Geometry check sheet. Reference: the model listing, model coordinates, mm. A direction names the side the tool comes from. Round coordinates to 2 decimals unless told otherwise and drop trailing zeros. Order: outer loops, then holes, each group sorted by start corner. A loop starts at its lowest first (then second) coordinate and runs counter-clockwise, first axis right, second up. Notation, with made-up numbers: (51, 5.25) - (62, 5.25) arc R32 cw to (62, 39.25) - close; hole circle Ø8 at (46, -2). An arc over 180 degrees is marked (long way). Write each question's results on one line, items separated by ' | '.
Autodesk Inventor part; units mm, degrees
ref_plane "YZ Plane" through (0, 0, 0) normal (1, 0, 0) x (0, 1, 0)
ref_plane "XZ Plane" through (0, 0, 0) normal (0, 1, 0) x (-1, 0, 0)
ref_plane "XY Plane" through (0, 0, 0) normal (0, 0, 1) x (1, 0, 0)
sketch "Sketch1" plane through (0, 0, 0) normal (0, 0, 1) x (1, 0, 0)
  circle A0 centre (0, 0) radius 1
  dimension "d0" = 2
extrude "Extrusion1" add sketch "Sketch1" along normal blind 30
ref_plane "Work Plane1" through (0, 0, 23) normal (0, 0, 1) x (1, 0, 0)
ref_plane "Work Plane2" through (0, 0, 7) normal (0, 0, -1) x (-1, 0, 0)
sketch "Sketch2" plane through (0, 0, 23) normal (0, 0, 1) x (1, 0, 0)
  circle A0 centre (0, 0) radius 1
  line L0 (1, 0) -> (-1, 0)
  line L1 (-1, 0) -> (-1, 26)
  line L2 (-1, 26) -> (1, 26)
  line L3 (1, 26) -> (1, 0)
  dimension "d7" = 26
extrude "Extrusion2" add sketch "Sketch2" against normal up to surface (16 mm away) contours A0 L1 L2 L3
sketch "Sketch3" plane through (1, 0, 23) normal (1, 0, 0) x (0, 0, -1)
  line L0 (16, 0) -> (16, 26)
  line L1 (0, 26) -> (16, 26)
  line L2 (0, 0) -> (0, 26)
  line L3 (16, 0) -> (0, 0)
  line L4 (0, 26) -> (-7, 26)
  line L5 (-7, 26) -> (-7, 4.5)
  line L6 (-7, 4.5) -> (0, 4.5)
  line L7 (0, 4.5) -> (0, 26)
  line L8 (16, 0) -> (16, 26)
  line L9 (16, 26) -> (23, 26)
  line L10 (23, 26) -> (23, 4.5)
  line L11 (23, 4.5) -> (16, 4.5)
  line L12 (16, 4.5) -> (16, 26)
  line L13 (23, -1) -> (23, 1)
  line L14 (-7, 1) -> (-7, -1)
  line L15 (16, 0) -> (0, 0)
  line L16 (16, 0) -> (16, 0)
  line L17 (16, 0) -> (0, 0)
  line L18 (0, 0) -> (0, 0)
  point P0 (23, 0)
  point P1 (19.5, 4.5)
  point P2 (-3.5, 4.5)
  point P3 (23, 0)
  point P4 (23, 15.25)
  point P5 (-7, 15.25)
  point P6 (-7, 0)
  dimension "d10" = 3.5
extrude "Extrusion3" add sketch "Sketch3" against normal up to surface (2 mm away) contours L0 L9 L10 L11 | L6 L5 L4 L2
properties part number "gpsDoor"
(1) Draft check along Y on faces 1 (the face through (0, 15, 0)), 2 (the face through (0, 4.5, 3)), 3 (the face through (0, 26, 15)). Enter one of: released by +Y, released by -Y, zero draft, split by the parting line, or undercut.
Answers follow:
face 1: zero draft | face 2: undercut | face 3: released by +Y
(2) Access from +Z, -Z, +X, -X, +Y, -Y to the whole of each face (thin tool, end or side, straight path). Record for faces 4 (the face through (0, 4.5, 27)), 5 (the face through (0, -1, 15)), 6 (the face through (-1, 13, 15)).
Answers follow:
face 4: +Z, +X, -X | face 5: none | face 6: +Z, -Z, -X, +Y, -Y
(3) Depth check by flat-ended pin: pin 1 Ø1 at (x, y) = (0, 2.5) entering from -Z. Enter the tip coordinate at first touch or a pass-through.
Answers follow:
pin 1: z = 7
(4) Material ranges on line 1 (Y direction, x = -0.8, z = 28.5); line 2 (Y direction, x = -0.15, z = 4); line 3 (Z direction, x = 0.85, y = 1.5), recorded low to high.
Answers follow:
line 1: -0.6 to 0.6, 4.5 to 26 | line 2: -0.99 to 0.99, 4.5 to 26 | line 3: 7 to 23
(5) Section check B-B (z = 24.5). Record the cut outline in (x, y).
Answers follow:
outline: circle Ø2 at (0, 0); (-1, 4.5) - (1, 4.5) - (1, 26) - (-1, 26) - close
(6) Section check A-A (x = 0). Record the cut outline in (y, z), then the cut area to 3 significant figures.
Answers follow:
outline: (-1, 0) - (1, 0) - (1, 7) - (4.5, 7) - (4.5, 0) - (26, 0) - (26, 30) - (4.5, 30) - (4.5, 23) - (1, 23) - (1, 30) - (-1, 30) - close | area: 761 mm²
